Geometry: final body of the model. Coordinates: model frame, mm. Coordinates: 2 decimals unless noted, no trailing zeros. Order: outer loops, then holes, each group sorted by start corner. A loop starts at its lowest first (then second) coordinate and runs counter-clockwise, first axis right, second up. Notation, with made-up numbers: M -34.5,-27 L 18.5,-27 A8 cw 18.5,-12 Z; hole C 11.5,53 d4. An arc over 180 degrees is marked long. Use CSV: the item, a comma, the result in double quotes. Start each with the question number.
Q1. Section query D-D, the plane z = 21. Output: boundary loops of the cut face in (x, y), and give its area (3 significant figures).
Q2. Section query B-B, the plane z = 0. Output: boundary loops of the cut face in (x, y).
Q3. Mould query, pull axis X, two halves, no side actions, for faces 1 (the face through (0, 1, -3)), 2 (the face through (8.196, 1.014, 23.289)), 3 (the face through (-8.289, 1.014, 23.196)), 4 (the face through (0, 1, -25)). Classes: +X half, -X half, draft (parallel to the pull), parting line (faces both ways), or undercut.
Q4. Section query C-C, the plane y = 1.6. Output: boundary loops of the cut face in (x, z).
Q5. Section query A-A, the plane x = 0. Output: boundary loops of the cut face in (y, z), and give its area (3 significant figures).
Q6. Ray query, probe 1 along Z at (x, y) = (0, 0.65); probe 2 along X at (y, z) = (1.3, 0); probe 3 along Z at (x, y) = (-2.75, 0.9). Return the intervals inside material, ascending.
Autodesk Inventor part; units mm, degrees
ref_plane "YZ Plane" through (0, 0, 0) normal (1, 0, 0) x (0, 1, 0)
ref_plane "XZ Plane" through (0, 0, 0) normal (0, 1, 0) x (-1, 0, 0)
ref_plane "XY Plane" through (0, 0, 0) normal (0, 0, 1) x (1, 0, 0)
sketch "草圖1" plane through (0, 0, 0) normal (0, 1, 0) x (-1, 0, 0)
  line L0 (10, 25) -> (-10, 25)
  line L1 (-10, 25) -> (-10, -25)
  line L2 (-10, -25) -> (10, -25)
  line L3 (10, -25) -> (10, 25)
  line L4 (10, 25) -> (-10, -25) construction
  line L5 (-10, 25) -> (10, -25) construction
  point P0 (0, 0)
  dimension "d0" = 20
  dimension "d1" = 50
extrude "平板1" add sketch "草圖1" along normal blind 2
fillet "轉角外圓角1" radius 6 4 edges at (10, 1, 25) (-10, 1, 25) (-10, 1, -25) (10, 1, -25)
sketch "草圖4" plane through (0, 2, 0) normal (0, 1, 0) x (1, 0, 0)
  point P0 (0, 0)
  point P1 (0, 0)
hole "孔2" at (0, 2, 0) direction (0, -1, 0) diameter 6 end through all
equation "\"d18\" = 厚度"
equation "\"d2\" = 厚度"
equation "\"折彎半徑\" = 厚度"
equation "\"折彎離隙寬度\" = 厚度"
equation "\"折彎離隙深度\" = 0.5 * 厚度"
equation "\"轉角離隙大小\" = 4 * 厚度"
equation "\"最小剩餘\" = 2 * 厚度"
equation "\"轉移半徑\" = 折彎半徑"
equation "\"Jacobi半徑大小\" = 折彎半徑"
equation "\"間隙大小\" = 厚度"
properties part number "底部外殼固定板金"
Responses:
1,outline,"M -9.66,0 L 9.66,0 L 9.66,2 L -9.66,2 Z"
1,area,"38.6 mm²"
2,outline,"M -10,0 L -3,0 L -3,2 L -10,2 Z; M 3,0 L 10,0 L 10,2 L 3,2 Z"
3,face 1,"undercut"
3,face 2,"+X half"
3,face 3,"-X half"
3,face 4,"draft"
4,outline,"M -10,-19 A6 ccw -4,-25 L 4,-25 A6 ccw 10,-19 L 10,19 A6 ccw 4,25 L -4,25 A6 ccw -10,19 Z; hole C 0,0 d6"
5,outline,"M 0,-25 L 2,-25 L 2,-3 L 0,-3 Z; M 0,3 L 2,3 L 2,25 L 0,25 Z"
5,area,"88.0 mm²"
6,probe 1,"z = -25 to -3, 3 to 25"
6,probe 2,"x = -10 to -3, 3 to 10"
6,probe 3,"z = -25 to -1.2, 1.2 to 25"
